Here's how the part is built. I have some questions about the finished solid (model axes, mm). Face numbers are marked on the shaded views. A direction names the side the tool comes from. Round coordinates to 2 decimals unless told otherwise and drop trailing zeros. Loops run counter-clockwise (first coordinate to the right, second up) from the corner with the lowest first, then second, coordinate; pieces in that order, holes last. Notation, with made-up numbers: M 10,27 L 52,27 A10 cw 52,38 Z; hole C 33.5,28.5 d11. An arc over 180 degrees is marked long. Answer as a JSON object with one key per item and string values.
from build123d import *

# Parameters (mm, degrees)
SKETCH1_R           = 5
SKETCH1_R_2         = 2.5
BOSS_EXTRUDE1_DEPTH = 18
SKETCH2_R           = 3.7
SKETCH2_R_2         = 2.5
CUT_EXTRUDE1_DEPTH  = 3.3
CUT_EXTRUDE2_START  = -14.7
SKETCH2_2_R         = 3.7
SKETCH2_2_R_2       = 2.5
CUT_EXTRUDE2_DEPTH  = 3.3


with BuildPart() as part:
    # Sketch1 → Boss-Extrude1 (new body)
    with BuildSketch(Plane(origin=(0, 0, 0), x_dir=(1, 0, 0), z_dir=(0, 1, 0))):
        with Locations(Location((0, 0, 0), (0, 0, 270))):
            Circle(SKETCH1_R)
        with Locations(Location((0, 0, 0), (0, 0, 270))):
            Circle(SKETCH1_R_2, mode=Mode.SUBTRACT)
    extrude(amount=BOSS_EXTRUDE1_DEPTH)

    # Sketch2 → Cut-Extrude1 (cut)
    with BuildSketch(Plane.XZ):
        with Locations(Location((0, 0, 0), (0, 0, 270))):
            Circle(SKETCH2_R)
        with Locations(Location((0, 0, 0), (0, 0, 270))):
            Circle(SKETCH2_R_2, mode=Mode.SUBTRACT)
    extrude(amount=-CUT_EXTRUDE1_DEPTH, mode=Mode.SUBTRACT)

    # Sketch2<2> → Cut-Extrude2 (cut)
    with BuildSketch(Plane.XZ.offset(CUT_EXTRUDE2_START)):
        with Locations(Location((0, 0, 0), (0, 0, 270))):
            Circle(SKETCH2_2_R)
        with Locations(Location((0, 0, 0), (0, 0, 270))):
            Circle(SKETCH2_2_R_2, mode=Mode.SUBTRACT)
    extrude(amount=-CUT_EXTRUDE2_DEPTH, mode=Mode.SUBTRACT)


solid = part.part
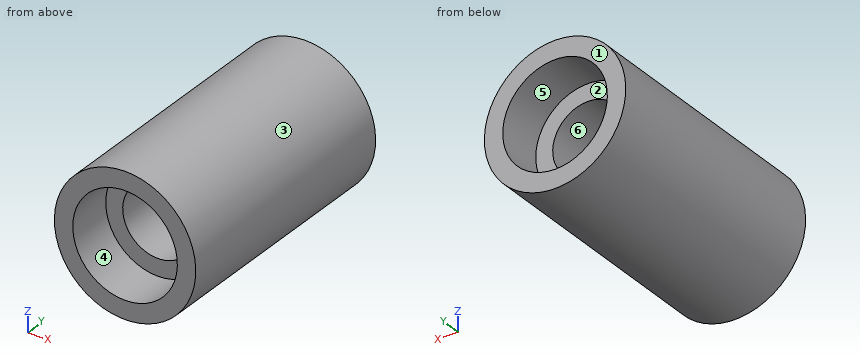
Item 1: On a 3-axis mill with a long thin cutter (end or side, diameter ignored), from which of +Z, -Z, +X, -X, +Y, -Y can I reach the whole of each face in a straight line? I mean the marked faces 4, 5 and 6. Say none if no direction works.
Resolved:
{"face 4": "-Y", "face 5": "+Y", "face 6": "+Y, -Y"}
Item 2: Please list where these lines run through material, in increasing order: probe 1 along X at (y, z) = (17.2, 0); probe 2 along X at (y, z) = (12.25, 0); probe 3 along Y at (x, z) = (-0.75, 2.5). Write a range as from..to.
Resolved:
{"probe 1": "-5..-3.7, 3.7..5", "probe 2": "-5..-2.5, 2.5..5", "probe 3": "3.3..14.7"}
Item 3: If we mould it in two halves opening along X, with no side actions, what happens to the marked faces 1, 2 and 3? For each: pulls with the +X half, pulls with the -X half, needs draft (parallel to the pull), parting line crosses it, or undercut.
Resolved:
{"face 1": "needs draft", "face 2": "undercut", "face 3": "parting line crosses it"}
Item 4: I want a section at A-A, the plane x = 0. Please give me the cut outline in (y, z), then the cut area to 3 significant figures.
Resolved:
{"outline": "M 0,-5 L 18,-5 L 18,-3.7 L 14.7,-3.7 L 14.7,-2.5 L 3.3,-2.5 L 3.3,-3.7 L 0,-3.7 Z; M 0,3.7 L 3.3,3.7 L 3.3,2.5 L 14.7,2.5 L 14.7,3.7 L 18,3.7 L 18,5 L 0,5 Z", "area": "74.2 mm²"}
Item 5: I'm going to push flat-ended pins straight in: pin 1 Ø6 at (x, z) = (0.5, 1.5) entering from -Y; pin 2 Ø1.5 at (x, z) = (1.5, 0.5) entering from -Y; pin 3 Ø3 at (y, z) = (2, 2.5) entering from -X; pin 4 Ø1.5 at (y, z) = (6, -2.5) entering from -X. Where does each tip first touch, or does it pass through?
Resolved:
{"pin 1": "y = 0", "pin 2": "through", "pin 3": "x = -4.9", "pin 4": "x = -4.68"}
Item 6: I want a section at C-C, the plane y = 5.25. Please give me the cut outline in (x, z).
Resolved:
{"outline": "C 0,0 d10; hole C 0,0 d5"}
Item 7: I want a section at B-B, the plane z = 0.25. Please give me the cut outline in (x, y).
Resolved:
{"outline": "M -4.99,0 L -3.69,0 L -3.69,3.3 L -2.49,3.3 L -2.49,14.7 L -3.69,14.7 L -3.69,18 L -4.99,18 Z; M 2.49,3.3 L 3.69,3.3 L 3.69,0 L 4.99,0 L 4.99,18 L 3.69,18 L 3.69,14.7 L 2.49,14.7 Z"}
Item 8: I want a section at D-D, the plane z = -3.25. Please give me the cut outline in (x, y).
Resolved:
{"outline": "M -3.8,0 L -1.77,0 L -1.77,3.3 L 1.77,3.3 L 1.77,0 L 3.8,0 L 3.8,18 L 1.77,18 L 1.77,14.7 L -1.77,14.7 L -1.77,18 L -3.8,18 Z"}
